Design review of the part built by this model. Coordinates are the model's own, in mm. Round coordinates to 2 decimals unless told otherwise and drop trailing zeros. Order: outer loops, then holes, each group sorted by start corner. A loop starts at its lowest first (then second) coordinate and runs counter-clockwise, first axis right, second up. Notation, with made-up numbers: M 8,29.5 L 12,29.5 A26 cw 12,64.5 Z; hole C -5.5,-31 d4. An arc over 180 degrees is marked long. Write each question's results on one line, items separated by ' | '. Start each with the question number.
Item 1: Take a section at B-B, the plane y = 20. Write out the cut boundary in (x, z).
Item 2: Wall thickness on line 1 (Y direction, x = 0, z = 1.4); line 2 (Y direction, x = 4.5, z = 1.9); line 3 (X direction, y = 16, z = 2.4): over which ranges is each line inside the solid? List them lowest first. Write a range as [from, to].
Item 3: Take a section at A-A, the plane x = 0. Write out the cut boundary in (y, z).
Item 4: Take a section at C-C, the plane z = 1.05. Write out the cut boundary in (x, y).
```python
from build123d import *

# Parameters (mm, degrees)
SZKIC1_W                    = 50
SZKIC1_H                    = 80
DODANIE_WYCI_GNI_CIE1_DEPTH = 3
OTW_R_GWINTOWANY_M121_D     = 10.2
OTW_R_GWINTOWANY_M121_DEPTH = 32.75
OTW_R_GWINTOWANY_M121_TIP   = 3.064389157


with BuildPart() as part:
    # Szkic1 → Dodanie-wyciągnięcie1 (new body)
    with BuildSketch(Plane.XY):
        Rectangle(SZKIC1_W, SZKIC1_H)
    extrude(amount=DODANIE_WYCI_GNI_CIE1_DEPTH)

    # Otwór gwintowany M121
    with Locations(Plane.XY.offset(3)):
        with Locations((0, 20)):
            Hole(OTW_R_GWINTOWANY_M121_D / 2, depth=OTW_R_GWINTOWANY_M121_DEPTH)
            with Locations((0, 0, -(OTW_R_GWINTOWANY_M121_DEPTH + OTW_R_GWINTOWANY_M121_TIP / 2))):  # 118° drill point
                Cone(0, OTW_R_GWINTOWANY_M121_D / 2, OTW_R_GWINTOWANY_M121_TIP, mode=Mode.SUBTRACT)


solid = part.part
```
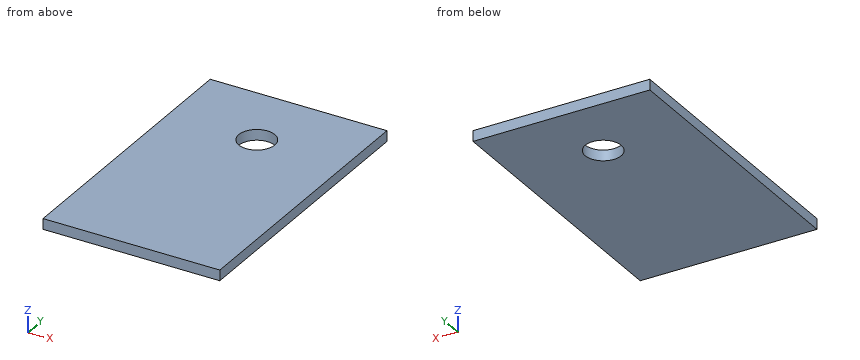
Results list:
1) outline: M -25,0 L -5.1,0 L -5.1,3 L -25,3 Z; M 5.1,0 L 25,0 L 25,3 L 5.1,3 Z
2) line 1: [-40, 14.9], [25.1, 40] | line 2: [-40, 17.6], [22.4, 40] | line 3: [-25, -3.16], [3.16, 25]
3) outline: M -40,0 L 14.9,0 L 14.9,3 L -40,3 Z; M 25.1,0 L 40,0 L 40,3 L 25.1,3 Z
4) outline: M -25,-40 L 25,-40 L 25,40 L -25,40 Z; hole C 0,20 d10.2
